Autodesk Inventor part; units mm, degrees
ref_plane "YZ Plane" through (0, 0, 0) normal (1, 0, 0) x (0, 1, 0)
ref_plane "XZ Plane" through (0, 0, 0) normal (0, 1, 0) x (-1, 0, 0)
ref_plane "XY Plane" through (0, 0, 0) normal (0, 0, 1) x (1, 0, 0)
sketch "Sketch1" plane through (0, 0, 0) normal (0, 0, 1) x (1, 0, 0)
  line L0 (-608.75, -609.5) -> (608.75, 609.5) construction
  line L1 (608.75, -609.5) -> (-608.75, 609.5) construction
  line L2 (-605.75, 606.5) -> (605.75, 606.5)
  line L3 (605.75, 606.5) -> (605.75, -606.5)
  line L4 (605.75, -606.5) -> (-605.75, -606.5)
  line L5 (-605.75, -606.5) -> (-605.75, 606.5)
  point P0 (0, 0)
  dimension "d0" = 1217.5
  dimension "d1" = 1219
extrude "Extrusion1" add sketch "Sketch1" along normal blind 1025
sketch "Sketch2" plane through (605.75, -606.5, 0) normal (1, 0, 0) x (0, 0, -1)
  line L0 (0, 0) -> (-1025, 0) construction
  line L1 (-639, 0) -> (-639, 1213) construction
  line L2 (0, 1213) -> (-1025, 1213) construction
  line L3 (-364, 0) -> (-364, 1204) construction
  line L4 (-89, 0) -> (-89, 1213) construction
  line L5 (-1025, 0) -> (-1025, 1213)
  line L6 (-1025, 122.5) -> (0, 122.5) construction
  line L7 (0, 0) -> (0, 1213) construction
  line L8 (-1025, 364.5) -> (0, 364.5) construction
  line L9 (-1025, 606.5) -> (0, 606.5) construction
  line L10 (-1025, 848.5) -> (0, 848.5) construction
  line L11 (-1025, 1090.5) -> (0, 1090.5) construction
  point P0 (0, 606.5)
  point P1 (-639, 1090.5)
  point P2 (-364, 1090.5)
  point P3 (-89, 1090.5)
  point P4 (-89, 848.5)
  point P5 (-89, 606.5)
  point P6 (-89, 364.5)
  point P7 (-89, 122.5)
  point P8 (-364, 122.5)
  point P9 (-364, 364.5)
  point P10 (-364, 606.5)
  point P11 (-364, 848.5)
  point P12 (-639, 848.5)
  point P13 (-639, 606.5)
  point P14 (-639, 364.5)
  point P15 (-639, 122.5)
  dimension "d5" = 386
  dimension "d6" = 275
  dimension "d7" = 275
  dimension "d8" = 122.5
  dimension "d9" = 242
  dimension "d10" = 242
  dimension "d11" = 242
  dimension "d12" = 242
  dimension "d13" = 122.5
sketch "Sketch3" plane through (-605.75, 606.5, 0) normal (0, 1, 0) x (1, 0, 0)
  line L0 (1211.5, -639) -> (0, -639) construction
  line L1 (0, 0) -> (0, -1025) construction
  line L2 (1211.5, -364) -> (7.5, -364) construction
  line L3 (1211.5, -89) -> (0, -89) construction
  line L4 (0, -1025) -> (1211.5, -1025) construction
  line L5 (122.5, -1025) -> (122.5, 0) construction
  line L6 (0, 0) -> (1211.5, 0) construction
  line L7 (364.5, -1000) -> (364.5, 0) construction
  line L8 (606.5, -1000) -> (606.5, 0) construction
  line L9 (848.5, -1025) -> (848.5, 0) construction
  line L10 (1090.5, -1025) -> (1090.5, 0) construction
  line L11 (1211.5, 0) -> (1211.5, -1025)
  point P0 (605.75, 0)
  point P1 (122.5, -639)
  point P2 (122.5, -364)
  point P3 (122.5, -89)
  point P4 (364.5, -89)
  point P5 (364.5, -364)
  point P6 (364.5, -639)
  point P7 (606.5, -639)
  point P8 (848.5, -639)
  point P9 (1090.5, -639)
  point P10 (1090.5, -364)
  point P11 (1090.5, -89)
  point P12 (848.5, -89)
  point P13 (848.5, -364)
  point P14 (606.5, -364)
  point P15 (606.5, -89)
  dimension "d14" = 121
  dimension "d15" = 242
  dimension "d16" = 242
  dimension "d17" = 242
  dimension "d18" = 242
  dimension "d19" = 122.5
shell "Shell1" thickness 1.5 removed faces 2 at (-201.9167, 202.1667, 0) at (-201.9167, 202.1667, 1025)
hole "Hole1" at (605.75, -484, 639) at (605.75, -242, 639) at (605.75, 0, 639) at (605.75, 242, 639) at (605.75, 484, 639) at (605.75, 484, 364) at (605.75, 242, 364) at (605.75, 0, 364) at (605.75, -242, 364) at (605.75, -484, 364) at (605.75, -484, 89) at (605.75, -242, 89) at (605.75, 0, 89) at (605.75, 242, 89) at (605.75, 484, 89) direction (-1, 0, 0) diameter 3 end through all
hole "Hole2" at (-483.25, 606.5, 639) at (-483.25, 606.5, 364) at (-483.25, 606.5, 89) at (-241.25, 606.5, 89) at (-241.25, 606.5, 364) at (-241.25, 606.5, 639) at (0.75, 606.5, 639) at (242.75, 606.5, 639) at (484.75, 606.5, 639) at (484.75, 606.5, 364) at (484.75, 606.5, 89) at (242.75, 606.5, 89) at (242.75, 606.5, 364) at (0.75, 606.5, 364) at (0.75, 606.5, 89) direction (0, -1, 0) diameter 3 end through all
properties part number "Entrance"
Could you check a few things on this model? Use its own coordinates, in mm. A direction names the side the tool comes from. Give positions to 0.01 mm unless a question says otherwise; leave off trailing zeros. Order: outer loops, then holes, each group sorted by start corner. A loop starts at its lowest first (then second) coordinate and runs counter-clockwise, first axis right, second up.
1. Suppose I cut it at A-A (y = -32.5). Write out the boundary of the cut face in (x, z), plus the area to 4 significant figures.
Answers below:
outline: (-605.75, 0) - (-604.25, 0) - (-604.25, 1025) - (-605.75, 1025) - close; (604.25, 0) - (605.75, 0) - (605.75, 1025) - (604.25, 1025) - close
area: 3,075 mm2
2. Thinking about a two-plate mould opening in X: for faces 3 (the flat face through (-8, 606.5, 505)), 4 (the flat face through (-605.75, -8, 505)), 5 (the flat face through (-604.25, -8, 505)), which applies, +X half, -X half, draft (parallel to the pull), parting line (faces both ways), or undercut?
Answers below:
face 3: draft
face 4: -X half
face 5: undercut
3. Suppose I cut it at B-B (z = 177). Write out the boundary of the cut face in (x, y), plus the area to 3 significant figures.
Answers below:
outline: (-605.75, -606.5) - (605.75, -606.5) - (605.75, 606.5) - (-605.75, 606.5) - close; hole (-604.25, -605) - (604.25, -605) - (604.25, 605) - (-604.25, 605) - close
area: 7,260 mm2
4. Suppose I cut it at C-C (x = 306). Write out the boundary of the cut face in (y, z).
Answers below:
outline: (-606.5, 0) - (-605, 0) - (-605, 1025) - (-606.5, 1025) - close; (605, 0) - (606.5, 0) - (606.5, 1025) - (605, 1025) - close
5. For pin 1 (2.5 mm diameter, centred on y = 0, z = 639, fed in from -X), with a flat end and sliding along its axis, tell me the tip position at first contact or that it passes through.
Answers below:
pin 1: passes through
6. Which directions (+Z, -Z, +X, -X, +Y, -Y) give clear straight access to the entire face, cutting with the end or side of a thin tool? Please do faces 1 (the flat face through (8, -606.5, 505)), 2 (the flat face through (-8, 605, 505)).
Answers below:
face 1: +Z, -Z, +X, -X, -Y
face 2: +Z, -Z
7. I need wall thicknesses on L1, parallel to Y at x = 605.15, z = 89; L2, parallel to X at y = 605.3, z = 364; L3, parallel to Z at x = 242.75, y = 605.9. Which ranges of each line are inside material? Lowest first, please.
Answers below:
L1: y = -606.5 to -485.5, -482.5 to -243.5, -240.5 to -1.5, 1.5 to 240.5, 243.5 to 482.5, 485.5 to 606.5
L2: x = -605.75 to -484.75, -481.75 to -242.75, -239.75 to -0.75, 2.25 to 241.25, 244.25 to 483.25, 486.25 to 605.75
L3: z = 0 to 87.5, 90.5 to 362.5, 365.5 to 637.5, 640.5 to 1025
